```python
from build123d import *

# Parameters (mm, degrees)
F2_R     = 2.54
F4_D     = 14.6812
F4_DEPTH = 12.7
F4_TIP   = 4.41067746
F5_SIZE  = 1.27
F6_SIZE  = 0.762


# Not quite as in the source:
# - a fillet or chamfer that OpenCascade refuses, or shapes differently, is made with other operations: its cross-section is extruded or revolved along the edge and cut away or added


with BuildPart() as f1:
    # F0 (on Front) → F1 (revolve)
    with BuildSketch(Plane.XZ):
        with BuildLine():
            ThreePointArc((-69.7489041133, -10.16), (-70.3007351719, -5.093315157), (-70.485, 0))
            Line((-70.485, 0), (-80.645, 0))
            Line((-80.645, 0), (-80.645, -10.16))
            Line((-80.645, -10.16), (-69.7489041133, -10.16))
        make_face()
        with BuildLine():
            ThreePointArc((69.215, 0), (0, -69.215), (-69.215, 0))
            Line((-69.215, 0), (-70.485, 0))
            ThreePointArc((-70.485, 0), (-70.3007351719, -5.093315157), (-69.7489041133, -10.16))
            ThreePointArc((-69.7489041133, -10.16), (-48.4655816688, -51.1783413028), (-6.35, -70.1983812135))
            ThreePointArc((-6.35, -70.1983812135), (-3.1782326193, -70.4133088444), (0, -70.485))
            ThreePointArc((0, -70.485), (3.1782326193, -70.4133088444), (6.35, -70.1983812135))
            ThreePointArc((6.35, -70.1983812135), (52.0370780069, -47.5423783324), (70.485, 0))
            Line((70.485, 0), (69.215, 0))
        make_face()
        with BuildLine():
            ThreePointArc((0, -70.485), (-3.1782326193, -70.4133088444), (-6.35, -70.1983812135))
            Line((-6.35, -70.1983812135), (-6.35, -72.517))
            Line((-6.35, -72.517), (0, -72.517))
            Line((0, -72.517), (0, -70.485))
        make_face()
        with BuildLine():
            Line((6.35, -72.517), (6.35, -70.1983812135))
            ThreePointArc((6.35, -70.1983812135), (3.1782326193, -70.4133088444), (0, -70.485))
            Line((0, -70.485), (0, -72.517))
            Line((0, -72.517), (6.35, -72.517))
        make_face()
    revolve(axis=Axis((-35.2425, 0, 0), (-1, 0, 0)))

    # F2
    f2_edges = [f1.edges().sort_by_distance(p)[0] for p in [
        (-69.748904, 0, 10.16),
    ]]
    fillet(f2_edges, radius=F2_R)

    # F4
    with Locations(Plane(origin=(-80.645, 0, 0), x_dir=(0, -1, 0), z_dir=(-1, 0, 0))):
        with Locations((0, 0)):
            Hole(F4_D / 2, depth=F4_DEPTH)
            with Locations((0, 0, -(F4_DEPTH + F4_TIP / 2))):  # 118° drill point
                Cone(0, F4_D / 2, F4_TIP, mode=Mode.SUBTRACT)

    # F5
    f5_edges = [f1.edges().sort_by_distance(p)[0] for p in [
        (-80.645, 0, 10.16),
    ]]
    chamfer(f5_edges, length=F5_SIZE)

    # F6
    f6_edges = [f1.edges().sort_by_distance(p)[0] for p in [
        (-6.35, 0, 72.517),
        (6.35, 0, 72.517),
    ]]
    chamfer(f6_edges, length=F6_SIZE)

    # F7: fillet of radius 2.032 on 2 edges, made by hand

    # F7_s1 → F7_t2 (revolve)
    with BuildSketch(Plane.XZ):
        with BuildLine():
            ThreePointArc((-6.35, -71.755), (-6.9417364445, -70.5807921178), (-8.1285337342, -70.0147281958))
            ThreePointArc((-8.1285337342, -70.0147281958), (-7.2398492305, -70.1121944323), (-6.35, -70.1983812135))
            Line((-6.35, -70.1983812135), (-6.35, -71.755))
        make_face()
    revolve(axis=Axis((-6.35, 0, 0), (-1, 0, 0)))

    # F7_s3 → F7_t4 (revolve)
    with BuildSketch(Plane.XZ):
        with BuildLine():
            ThreePointArc((6.35, -71.755), (6.9417364445, -70.5807921178), (8.1285337342, -70.0147281958))
            ThreePointArc((8.1285337342, -70.0147281958), (7.2398492305, -70.1121944323), (6.35, -70.1983812135))
            Line((6.35, -70.1983812135), (6.35, -71.755))
        make_face()
    revolve(axis=Axis((6.35, 0, 0), (-1, 0, 0)))


solid = f1.part
```
CAD build for the part. Positions are in the model's coordinates, mm. Round coordinates to 2 decimals unless told otherwise and drop trailing zeros. Loops run counter-clockwise (first coordinate to the right, second up) from the corner with the lowest first, then second, coordinate; pieces in that order, holes last. Notation, with made-up numbers: M 37,-17.75 L 69,-17.75 A15 cw 69,-12.75 Z; hole C 73,67.25 d9. An arc over 180 degrees is marked long. Use a Markdown table: item, result. Add a question column.
(1) Pull direction Y, two halves, no side cores. Call faces 1 (the face through (-74.652, 7.002, 2.205)), 2 (the face through (-75.591, -10.074, 1.323)), 3 (the face through (-80.645, -7, -3)): +Y half, -Y half, draft (parallel to the pull), parting line (faces both ways), or undercut.
(2) Flat gauge pins, fed straight in: pin 1 (3 mm diameter, centred on x = -9, y = 44.5, fed in from -Z); pin 2 (8 mm diameter, centred on x = 24.5, z = -14, fed in from -Y); pin 3 (10 mm diameter, centred on x = 16, y = 17.5, fed in from -Z). Where does each tip first touch, or does it go through?
(3) Drill centre lines: line 1 (Y direction, x = -76.5, z = 0); line 2 (Y direction, x = 24, z = -13.5). Where is each one in solid material? Low to high.
(4) Cut at A-A (x = 48.5). Give the cut face in (y, z).
Geometry says:
| question | item | result |
|---|---|---|
| 1 | face 1 | undercut |
| 1 | face 2 | parting line |
| 1 | face 3 | draft |
| 2 | pin 1 | stops at z = -55.14 |
| 2 | pin 2 | stops at y = -66.19 |
| 2 | pin 3 | stops at z = -67.96 |
| 3 | line 1 | y = -10.16 to -7.34, 7.34 to 10.16 |
| 3 | line 2 | y = -64.88 to -63.5, 63.5 to 64.88 |
| 4 | outline | C 0,0 d102.29; hole C 0,0 d98.76 |
